Print and shaded views of the part. All mm, measured from the part's lowest x, y and z. Round coordinates to 2 decimals unless told otherwise and drop trailing zeros. Loops run counter-clockwise (first coordinate to the right, second up) from the corner with the lowest first, then second, coordinate; pieces in that order, holes last. Notation, with made-up numbers: (-1, 89.5) -> (44, 89.5) arc R25 ccw to (44, 103.5) -> close; hole circle Ø6 at (9, 22.5). An arc over 180 degrees is marked (long way). Use a Markdown table: item, result.
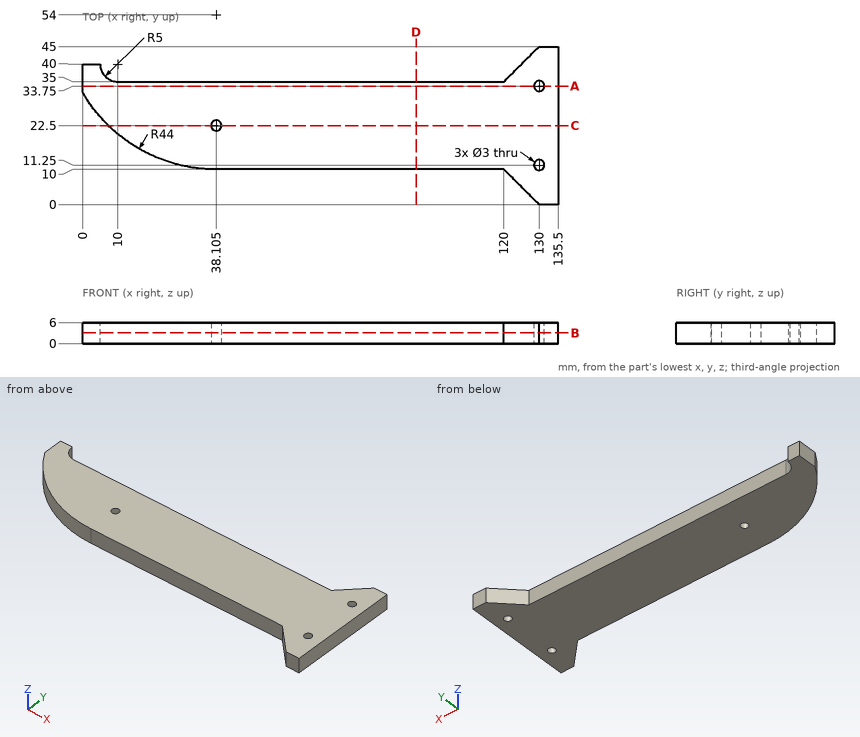
Q1. Band-saw the part on A-A, the plane y = 33.75. Give the cut face in (x, z).
Results list:
| item | result |
|---|---|
| outline | (0, 0) -> (128.5, 0) -> (128.5, 6) -> (0, 6) -> close; (131.5, 0) -> (135.5, 0) -> (135.5, 6) -> (131.5, 6) -> close |
Q2. Band-saw the part on C-C, the plane y = 22.5. Give the cut face in (x, z) (1 decimal), plus the area to 3 significant figures.
Results list:
| item | result |
|---|---|
| outline | (7.4, 0) -> (36.6, 0) -> (36.6, 6) -> (7.4, 6) -> close; (39.6, 0) -> (135.5, 0) -> (135.5, 6) -> (39.6, 6) -> close |
| area | 751 mm² |
Q3. Flat gauge pins, fed straight in: pin 1 (1.5 mm diameter, centred on x = 2, z = 4, fed in from +Y); pin 2 (3 mm diameter, centred on x = 96.5, z = 4.5, fed in from -Y); pin 3 (3.5 mm diameter, centred on x = 130, y = 11.25, fed in from +Z); pin 4 (3 mm diameter, centred on y = 6.5, z = 1.5, fed in from -X). Where does each tip first touch, or does it go through?
Results list:
| item | result |
|---|---|
| pin 1 | stops at y = 40 |
| pin 2 | stops at y = 10 |
| pin 3 | stops at z = 6 |
| pin 4 | stops at x = 122 |
Q4. Drill centre lines: L1, parallel to Y at x = 130, z = 3.8; L2, parallel to X at y = 25, z = 0.7; L3, parallel to Y at x = 98, z = 1.4. Where is each one in solid material? Low to high. Write a range as from..to.
Results list:
| item | result |
|---|---|
| L1 | y = 0..9.75, 12.75..32.25, 35.25..45 |
| L2 | x = 5.01..135.5 |
| L3 | y = 10..35 |
Q5. Band-saw the part on D-D, the plane x = 95. Give the cut face in (y, z).
Results list:
| item | result |
|---|---|
| outline | (10, 0) -> (35, 0) -> (35, 6) -> (10, 6) -> close |
Q6. Band-saw the part on B-B, the plane z = 3.05. Give the cut face in (x, y) (3 decimals).
Results list:
| item | result |
|---|---|
| outline | (0, 32) arc R44 ccw to (38.105, 10) -> (120, 10) -> (130, 0) -> (135.5, 0) -> (135.5, 45) -> (130, 45) -> (120, 35) -> (10, 35) arc R5 cw to (5, 40) -> (0, 40) -> close; hole circle Ø3 at (38.105, 22.5); hole circle Ø3 at (130, 11.25); hole circle Ø3 at (130, 33.75) |
